Verification items for the finished model (mm, model axes). Face numbers are marked on the shaded views. A direction names the side the tool comes from. Give positions to 0.01 mm unless a question says otherwise; leave off trailing zeros. Loops run counter-clockwise (first coordinate to the right, second up) from the corner with the lowest first, then second, coordinate; pieces in that order, holes last. Notation, with made-up numbers: M 81,-16 L 138,-16 A28 cw 138,11 Z; hole C 22.25,40.5 d3. An arc over 180 degrees is marked long. Put each result on its own line as item: value. Start each with the question number.
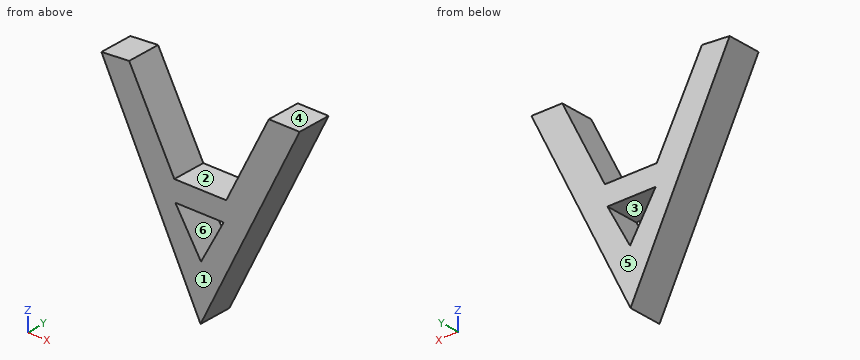
from build123d import *

# Parameters (mm, degrees)
F1_DEPTH = 25.4


with BuildPart() as f1:
    # F0 (on Front) → F1 (new body)
    with BuildSketch(Plane.XZ):
        Polygon((-53.987332, 76.514423), (-74.960828, 74.960828), (0, -75.737618), (74.960828, 75.737618), (51.656947, 75.737618), (19.419903, 11.651943), (-19.808304, 11.651943), align=None)
        Polygon((0.364124, -35.061012), (-19.031508, -3.495583), (17.477909, -3.495583), align=None, mode=Mode.SUBTRACT)
    extrude(amount=F1_DEPTH)


solid = f1.part
Q1. Go/stop test with flat-tipped pins: pin 1 (7.5 mm diameter, centred on x = -7, y = -9.5, fed in from -Z); pin 2 (1.5 mm diameter, centred on x = 56.5, y = -9.5, fed in from -Z); pin 3 (3 mm diameter, centred on x = 57, y = -20, fed in from -Z). Record where each tip stops, or that it passes through.
Q2. Cross-section at A-A, the plane y = -16.25. Record the boundary of the cut face in (x, z), then the cut area to 3 significant figures.
Q3. Cross-section at C-C, the plane x = 11. Record the boundary of the cut face in (y, z), then the cut area to 3 significant figures.
Q4. Cross-section at B-B, the plane z = 61. Record the boundary of the cut face in (x, y), then the cut area to 3 significant figures.
Q5. Cross-section at D-D, the plane x = -33. Record the boundary of the cut face in (y, z), then the cut area to 3 significant figures.
Q6. Scan lines: L1, parallel to X at y = -21.75, z = 15.5; L2, parallel to X at y = -23.25, z = 42; L3, parallel to Z at x = -11, y = -8.5. Record each from-to range of solid material in increasing order.
Q7. Set-up check for the marked faces 1 and 2: record each of +Z, -Z, +X, -X, +Y, -Y from which the full face is reachable in a straight line by a thin tool's end or side.
Q8. Release check for a two-part mould opening along Z. For the marked faces 3, 4, 5 and 6 record: pulls with the +Z half, pulls with the -Z half, needs draft (parallel to the pull), parting line crosses it, or undercut.
Ans:
1. pin 1: stops at z = -69.2
1. pin 2: stops at z = 36.92
1. pin 3: stops at z = 36.41
2. outline: M -74.96,74.96 L 0,-75.74 L 74.96,75.74 L 51.66,75.74 L 19.42,11.65 L -19.81,11.65 L -53.99,76.51 Z; hole M -19.03,-3.5 L 0.36,-35.06 L 17.48,-3.5 Z
2. area: 6,180 mm^2
3. outline: M -25.4,-53.51 L 0,-53.51 L 0,-15.44 L -25.4,-15.44 Z; M -25.4,-3.5 L 0,-3.5 L 0,11.65 L -25.4,11.65 Z
3. area: 1,350 mm^2
4. outline: M -68.02,-25.4 L -45.81,-25.4 L -45.81,0 L -68.02,0 Z; M 44.24,-25.4 L 67.67,-25.4 L 67.67,0 L 44.24,0 Z
4. area: 1,160 mm^2
5. outline: M -25.4,-9.4 L 0,-9.4 L 0,36.69 L -25.4,36.69 Z
5. area: 1,170 mm^2
6. L1: x = -45.38 to -21.84, 21.36 to 45.15
6. L2: x = -58.57 to -35.8, 34.69 to 58.27
6. L3: z = -53.62 to -16.57, -3.5 to 11.65
7. face 1: +Z, -Z, +X, -X, -Y
7. face 2: +Z, +Y, -Y
8. face 3: undercut
8. face 4: pulls with the +Z half
8. face 5: needs draft
8. face 6: undercut
